Could you check a few things on this model? Use its own coordinates, in mm. A direction names the side the tool comes from. Give positions to 0.01 mm unless a question says otherwise; leave off trailing zeros. Loops run counter-clockwise (first coordinate to the right, second up) from the corner with the lowest first, then second, coordinate; pieces in that order, holes last. Notation, with made-up numbers: (-22, -24) - (10, -24) arc R26 ccw to (10, -6) - close; hole circle Ø3 at (-6.75, 2). An arc over 180 degrees is marked (long way). One line per item, written item: value. Start each with the question number.
Q1. I want a section at C-C (z = -55.88). Please give me the cut outline in (x, y).
Q2. If I drill on line 1 (X direction, y = 21, z = -18); line 2 (Y direction, x = -2.5, z = -56); line 3 (Z direction, x = 9, y = -16.5), over which ranges is the centre line in solid material (lowest first)? Write a range as from..to.
Q3. If we mould it in two halves opening along Z, with no side actions, what happens to faces 3 (the face through (-18, -6, 0)), 4 (the face through (2.72, -17.51, -17.88)), 5 (the face through (-18, -6, -66.04))? For each: released by +Z, released by -Z, zero draft, split by the parting line, or undercut.
Q4. I want a section at D-D (x = 9). Please give me the cut outline in (y, z), then the cut area to 3 significant figures.
Q5. I want a section at A-A (z = -33.02). Please give me the cut outline in (x, y).
Q6. For faces 1 (the face through (-18.881, 7.289, -38.227)), 2 (the face through (5, -15.711, -33)), which set-ups out of +Z, -Z, +X, -X, +Y, -Y let a thin tool reach every point of the face, with its end or its side?
Q7. I want a section at B-B (y = 4). Please give me the cut outline in (x, z), then the cut area to 3 significant figures.
Q8. I'm going to push flat-ended pins straight in: P1, Ø20.5, axis at y = 16, z = -36, coming from the +X side; P2, Ø3, axis at x = -4.5, z = -46.5, coming from the +Y side. Where does each tip first touch, or does it pass through?
```python
from build123d import *

# Parameters (mm, degrees)
BOSS_EXTRUDE1_DEPTH = 66.04
FILLET1_R           = 1.27
FILLET3_R           = 5.08
SKETCH2_R           = 5.334
SKETCH2_R_2         = 4.064
CUT_EXTRUDE1_DEPTH  = 66.04
SKETCH3_R           = 5.334
CUT_EXTRUDE2_DEPTH  = 66.04


with BuildPart() as part:
    # Sketch1 → Boss-Extrude1 (new body)
    with BuildSketch(Plane.XY):
        Polygon((-20.634190635, 26.453063941), (-20.634190635, -19.266936059), (25.085809365, -19.266936059), (25.085809365, -15.710936059), (-17.078190635, -15.710936059), (-17.078190635, 26.453063941), align=None)
    extrude(amount=-BOSS_EXTRUDE1_DEPTH)

    # Fillet1
    fillet1_edges = [part.edges().sort_by_distance(p)[0] for p in [
        (-17.078190635, -15.710936059, -33.02),
    ]]
    fillet(fillet1_edges, radius=FILLET1_R)

    # Fillet3
    fillet3_edges = [part.edges().sort_by_distance(p)[0] for p in [
        (-20.634190635, -19.266936059, -33.02),
    ]]
    fillet(fillet3_edges, radius=FILLET3_R)

    # Sketch2 → Cut-Extrude1 (cut)
    with BuildSketch(Plane.ZY.offset(20.634190635)):
        with Locations(Location((-33.02, 6.133063941, 0), (0, 0, 270))):  # turned: the seam where the file's is
            Circle(SKETCH2_R)
        with Locations(Location((-55.88, 6.133063941, 0), (0, 0, 270))):  # turned: the seam where the file's is
            Circle(SKETCH2_R_2)
        with Locations(Location((-10.16, 6.133063941, 0), (0, 0, 270))):  # turned: the seam where the file's is
            Circle(SKETCH2_R_2)
    extrude(amount=-CUT_EXTRUDE1_DEPTH, mode=Mode.SUBTRACT)

    # Sketch3 → Cut-Extrude2 (cut)
    with BuildSketch(Plane(origin=(0, -19.266936059, 0), x_dir=(-1, 0, 0), z_dir=(0, -1, 0))):
        with Locations(Location((-4.765809365, 12.954, 0), (0, 0, 90))):  # turned: the seam where the file's is
            Circle(SKETCH3_R)
        with Locations(Location((-4.765809365, 53.34, 0), (0, 0, 90))):  # turned: the seam where the file's is
            Circle(SKETCH3_R)
    extrude(amount=-CUT_EXTRUDE2_DEPTH, mode=Mode.SUBTRACT)


solid = part.part
```
Worked answers:
1. outline: (-20.63, -14.19) arc R5.08 ccw to (-15.55, -19.27) - (0.08, -19.27) - (0.08, -15.71) - (-15.81, -15.71) arc R1.27 cw to (-17.08, -14.44) - (-17.08, 2.07) - (-20.63, 2.07) - close; (-20.63, 10.2) - (-17.08, 10.2) - (-17.08, 26.45) - (-20.63, 26.45) - close; (9.46, -19.27) - (25.09, -19.27) - (25.09, -15.71) - (9.46, -15.71) - close
2. line 1: x = -20.63..-17.08
2. line 2: y = -19.27..-15.71
2. line 3: z = -66.04..-56.58, -50.1..-16.2, -9.71..0
3. face 3: released by +Z
3. face 4: undercut
3. face 5: released by -Z
4. outline: (-19.27, -66.04) - (-15.71, -66.04) - (-15.71, -56.58) - (-19.27, -56.58) - close; (-19.27, -50.1) - (-15.71, -50.1) - (-15.71, -16.2) - (-19.27, -16.2) - close; (-19.27, -9.71) - (-15.71, -9.71) - (-15.71, 0) - (-19.27, 0) - close
4. area: 189 mm²
5. outline: (-20.63, -14.19) arc R5.08 ccw to (-15.55, -19.27) - (25.09, -19.27) - (25.09, -15.71) - (-15.81, -15.71) arc R1.27 cw to (-17.08, -14.44) - (-17.08, 0.8) - (-20.63, 0.8) - close; (-20.63, 11.47) - (-17.08, 11.47) - (-17.08, 26.45) - (-20.63, 26.45) - close
6. face 1: +X, -X
6. face 2: +Z, -Z, +X, +Y
7. outline: (-20.63, -66.04) - (-17.08, -66.04) - (-17.08, -59.34) - (-20.63, -59.34) - close; (-20.63, -52.42) - (-17.08, -52.42) - (-17.08, -37.91) - (-20.63, -37.91) - close; (-20.63, -28.13) - (-17.08, -28.13) - (-17.08, -13.62) - (-20.63, -13.62) - close; (-20.63, -6.7) - (-17.08, -6.7) - (-17.08, 0) - (-20.63, 0) - close
7. area: 151 mm²
8. P1: stops at x = -17.08
8. P2: stops at y = -15.71
